from build123d import *

# Parameters (mm, degrees)
SKETCH5_R           = 1.6
BOSS_EXTRUDE2_DEPTH = 2
SKETCH6_R           = 5.5
BOSS_EXTRUDE3_DEPTH = 14.5
FILLET1_R           = 1
SKETCH7_R           = 0.5
BOSS_EXTRUDE4_DEPTH = 0.6


with BuildPart() as part:
    # Sketch5 → Boss-Extrude2 (new body)
    with BuildSketch(Plane(origin=(0, 0, 0), x_dir=(1, 0, 0), z_dir=(0, 1, 0))):
        with BuildLine():
            Line((-11.250000051, -22.142785594), (-3.22490315, -22.142785594))
            ThreePointArc((-3.22490315, -22.142785594), (-5.1e-08, -27.342785594), (3.224903048, -22.142785594))
            Line((3.224903048, -22.142785594), (11.249999949, -22.142785594))
            ThreePointArc((11.249999949, -22.142785594), (24.240381006, -14.642785594), (24.240381006, 0.357214406))
            Line((24.240381006, 0.357214406), (20.227832555, 7.30715219))
            ThreePointArc((20.227832555, 7.30715219), (23.118713105, 12.700000199), (17.002929456, 12.892848208))
            Line((17.002929456, 12.892848208), (12.990381006, 19.842785992))
            ThreePointArc((12.990381006, 19.842785992), (-5.1e-08, 27.342785992), (-12.990381108, 19.842785992))
            Line((-12.990381108, 19.842785992), (-17.002929558, 12.892848208))
            ThreePointArc((-17.002929558, 12.892848208), (-23.118713208, 12.700000199), (-20.227832658, 7.30715219))
            Line((-20.227832658, 7.30715219), (-24.240381108, 0.357214406))
            ThreePointArc((-24.240381108, 0.357214406), (-24.240381108, -14.642785594), (-11.250000051, -22.142785594))
        make_face()
        with Locations((20.001021652, 10.900000199)):
            Circle(SKETCH5_R, mode=Mode.SUBTRACT)
        with Locations((-5.1e-08, -23.742785594)):
            Circle(SKETCH5_R, mode=Mode.SUBTRACT)
        with Locations((-20.001021754, 10.900000199)):
            Circle(SKETCH5_R, mode=Mode.SUBTRACT)
    extrude(amount=BOSS_EXTRUDE2_DEPTH)

    # Sketch6 → Boss-Extrude3 (add)
    with BuildSketch(Plane(origin=(0, 0, 0), x_dir=(1, 0, 0), z_dir=(0, 1, 0))):
        with Locations((-0.060025126, 12.462836141)):
            Circle(SKETCH6_R)
        with Locations((11.189974874, -7.022735444)):
            Circle(SKETCH6_R)
        with Locations((-11.310025126, -7.022735444)):
            Circle(SKETCH6_R)
    extrude(amount=BOSS_EXTRUDE3_DEPTH)

    # Fillet1
    fillet1_edges = [part.edges().sort_by_distance(p)[0] for p in [
        (-5.560025126, 14.5, -12.462836141),
        (5.689974874, 14.5, 7.022735444),
        (-16.810025126, 14.5, 7.022735444),
    ]]
    fillet(fillet1_edges, radius=FILLET1_R)

    # Sketch7 → Boss-Extrude4 (add)
    with BuildSketch(Plane(origin=(-18.334964206, 0, -10.58569652), x_dir=(-0.5, 0, 0.866025404), z_dir=(-0.866025404, 0, -0.5))):
        with Locations((-9.600955549, 1)):
            Circle(SKETCH7_R)
        with Locations((-7.600955549, 1)):
            Circle(SKETCH7_R)
    extrude(amount=BOSS_EXTRUDE4_DEPTH)


solid = part.part
Geometry check sheet. Reference: the model listing, model coordinates, mm. A direction names the side the tool comes from. Give positions to 0.01 mm unless a question says otherwise; leave off trailing zeros. Order: outer loops, then holes, each group sorted by start corner. A loop starts at its lowest first (then second) coordinate and runs counter-clockwise, first axis right, second up.
1. Scan lines: line 1 (X direction, y = 1.2, z = -10.9); line 2 (Z direction, x = 0, y = 1.4); line 3 (Y direction, x = -2, z = -1). Record each from-to range of solid material in increasing order.
Completed:
line 1: x = -23.6 to -21.6, -18.4 to 18.4, 21.6 to 23.6
line 2: z = -27.34 to 22.14, 25.34 to 27.34
line 3: y = 0 to 2
2. Sectioned sample at C-C (z = -1.5). Record the boundary of the cut face in (x, y).
Completed:
outline: (-23.58, 0) - (23.58, 0) - (23.58, 2) - (-23.58, 2) - close
3. Sectioned sample at B-B (y = 10). Record the boundary of the cut face in (x, z).
Completed:
outline: circle Ø11 at (-11.31, 7.02); circle Ø11 at (-0.06, -12.46); circle Ø11 at (11.19, 7.02)
4. Sectioned sample at A-A (z = -10.9). State how many separate pieces and enclosed holes the cut face has, then the cut area to 3 significant figures.
Completed:
separate pieces: 3
enclosed holes: 0
area: 213 mm2
5. Access from +Z, -Z, +X, -X, +Y, -Y to the whole of each face (thin tool, end or side, straight path). Record for faces 1 (the face through (-1.252, 7.67, -7.094)), 2 (the face through (22.262, 0.986, -3.784)), 3 (the face through (-21.271, 0.986, -9.926)).
Completed:
face 1: +Y
face 2: +X, +Y, -Y
face 3: +Y, -Y
6. Draft check along X on faces 4 (the face through (15.025, 0.986, -16.319)), 5 (the face through (7, 1, 22.143)), 6 (the face through (24.13, 0.99, 14.83)). Enter one of: pulls with the +X half, pulls with the -X half, needs draft (parallel to the pull), parting line crosses it, or undercut.
Completed:
face 4: undercut
face 5: needs draft
face 6: pulls with the +X half
7. Depth check by flat-ended pin: pin 1 (1.5 mm diameter, centred on x = 3, z = -10.5, fed in from -Y); pin 2 (6 mm diameter, centred on y = 8, z = -5, fed in from -X); pin 3 (0.6 mm diameter, centred on x = 6, y = 0.5, fed in from +Z); pin 4 (8 mm diameter, centred on y = 2.5, z = -16, fed in from -X). Enter the tip coordinate at first touch or a pass-through.
Completed:
pin 1: stops at y = 0
pin 2: stops at x = -3.27
pin 3: stops at z = 22.14
pin 4: stops at x = -23.42
8. Sectioned sample at D-D (z = -20.5). Record the boundary of the cut face in (x, y).
Completed:
outline: (-12.59, 0) - (12.59, 0) - (12.59, 2) - (-12.59, 2) - close
